Autodesk Inventor part; units mm, degrees
ref_plane "YZ Plane" through (0, 0, 0) normal (1, 0, 0) x (0, 1, 0)
ref_plane "XZ Plane" through (0, 0, 0) normal (0, 1, 0) x (-1, 0, 0)
ref_plane "XY Plane" through (0, 0, 0) normal (0, 0, 1) x (1, 0, 0)
sketch "Sketch1" plane through (0, 0, 0) normal (0, 0, 1) x (1, 0, 0)
  line L0 (-10.16, 6.415) -> (10.16, 6.415)
  line L1 (10.16, 6.415) -> (10.16, -6.415)
  line L2 (10.16, -6.415) -> (-10.16, -6.415)
  line L3 (-10.16, -6.415) -> (-10.16, 6.415)
  point P0 (0, 0)
  dimension "d0" = 20.32
  dimension "d1" = 10.16
  dimension "d2" = 12.83
  dimension "d3" = 6.415
extrude "Extrusion1" add sketch "Sketch1" along normal blind 6.35
sketch "Sketch2" plane through (0, 0, 0) normal (0, 0, -1) x (-1, 0, 0)
  line L0 (8.215, 7.24) -> (7.025, 7.24)
  line L1 (7.025, 7.24) -> (7.025, 5.59)
  line L2 (7.025, 5.59) -> (8.215, 5.59)
  line L3 (8.215, 5.59) -> (8.215, 7.24)
  line L4 (10.16, 6.415) -> (-10.16, 6.415)
  line L5 (10.16, -6.415) -> (10.16, 6.415)
  point P0 (0, 0)
  dimension "d6" = 1.65
  dimension "d7" = 0.825
  dimension "d8" = 1.19
  dimension "d9" = 1.945
extrude "Extrusion2" add sketch "Sketch2" against normal blind 1.27
pattern_linear "Rectangular Pattern1" count 7 spacing 2.54 along (1, 0, 0) of "Extrusion2"
mirror "Mirror1" about plane through (0, 0, 0) normal (0, 1, 0) of "Extrusion2", "Rectangular Pattern1"
properties part number "MC_BK377"
Can you work these out from the model? Positions are in its coordinate system, mm. A direction names the side the tool comes from. Coordinates: 2 decimals unless noted, no trailing zeros. Loops run counter-clockwise (first coordinate to the right, second up) from the corner with the lowest first, then second, coordinate; pieces in that order, holes last. Notation, with made-up numbers: M -2.75,30.25 L 45.25,30.25 A18 ccw 45.25,59.25 Z; hole C 18.25,25 d9. An arc over 180 degrees is marked long. Return JSON: item names as keys, results as strings. Group by question number.
Item 1: If I drill on L1, parallel to Y at x = -6.25, z = 5.25 (3 decimals), over which ranges is the centre line in solid material (lowest first)? Write a range as from..to.
Item 2: On a 3-axis mill with a long thin cutter (end or side, diameter ignored), from which of +Z, -Z, +X, -X, +Y, -Y can I reach the whole of each face in a straight line? I mean faces 4 (the flat face through (2.5, 6.8, 1.27)), 5 (the flat face through (0, 0, 0)), 6 (the flat face through (-1.945, -7, 1)), 7 (the flat face through (0.595, 7, 1)), 8 (the flat face through (-5, 7.24, 1)). Say none if no direction works.
Item 3: Imagine slicing it at B-B (z = 2). Please give me the cut outline in (x, y) (3 decimals).
Item 4: Thinking about a two-plate mould opening in X: for faces 1 (the flat face through (-5, -7.24, 1)), 2 (the flat face through (-5.675, -7, 1)), 3 (the flat face through (-8.215, 7, 1)), which applies, released by +X, released by -X, zero draft, split by the parting line, or undercut?
Item 5: Imagine slicing it at A-A (x = -8). Please give me the cut outline in (y, z) (3 decimals), and give its area (3 significant figures).
Item 6: Imagine slicing it at C-C (x = 6.25). Please give me the cut outline in (y, z) (3 decimals), and give its area (3 significant figures).
Item 7: I'm going to push flat-ended pins straight in: pin 1 Ø2 at (x, z) = (4.5, 5.5) entering from -Y (3 decimals); pin 2 Ø0.7 at (y, z) = (-6.5, 0.5) entering from -X; pin 3 Ø0.7 at (y, z) = (7, 1) entering from -X (3 decimals); pin 4 Ø0.9 at (x, y) = (0, 7) entering from +Z. Where does each tip first touch, or does it pass through?
Verdict:
{
 "1": {"L1": "y = -6.415..6.415"},
 "2": {"face 4": "+Z, +X, -X, +Y", "face 5": "-Z, +X, -X, +Y, -Y", "face 6": "+Z, -Z, -Y", "face 7": "+Z, -Z, +Y", "face 8": "+Z, -Z, +X, -X, +Y"},
 "3": {"outline": "M -10.16,-6.415 L 10.16,-6.415 L 10.16,6.415 L -10.16,6.415 Z"},
 "4": {"face 1": "zero draft", "face 2": "undercut", "face 3": "released by -X"},
 "5": {"outline": "M -7.24,0 L 7.24,0 L 7.24,1.27 L 6.415,1.27 L 6.415,6.35 L -6.415,6.35 L -6.415,1.27 L -7.24,1.27 Z", "area": "83.6 mm^2"},
 "6": {"outline": "M -6.415,0 L 6.415,0 L 6.415,6.35 L -6.415,6.35 Z", "area": "81.5 mm^2"},
 "7": {"pin 1": "stops at y = -6.415", "pin 2": "stops at x = -10.16", "pin 3": "stops at x = -8.215", "pin 4": "stops at z = 1.27"}
}
